Part model, mm, in its own coordinate system. A direction names the side the tool comes from. Round coordinates to 2 decimals unless told otherwise and drop trailing zeros. Order: outer loops, then holes, each group sorted by start corner. A loop starts at its lowest first (then second) coordinate and runs counter-clockwise, first axis right, second up. Notation, with made-up numbers: M 55.5,17 L 94.5,17 A11 ccw 94.5,26 Z; hole C 82,17 d4. An arc over 180 degrees is marked long. Write each question's results on one line, items separated by ' | '. Start each with the question number.
1. Two-plate mould, pull along Z, no slides. Class faces 6 (the face through (-74.289, -12.325, -74.196)), 7 (the face through (64, 0, 16)), 8 (the face through (77, 2, -1)): +Z half, -Z half, draft (parallel to the pull), parting line (faces both ways), or undercut.
2. Band-saw the part on C-C, the plane y = -59.5. List the corners of the cut face in (x, z), then the cut area to 3 significant figures.
3. Band-saw the part on A-A, the plane x = 0. List the corners of the cut face in (y, z).
4. Drop flat-ended pins along their axis: pin 1 Ø2 at (y, z) = (-39.5, 18) entering from +X; pin 2 Ø1.6 at (y, z) = (-7.5, 70.5) entering from -X; pin 3 Ø1 at (y, z) = (-13, 71) entering from +X. Give the stop position or say it passes through.
5. Probe L1, parallel to Z at x = 0, y = 1; L2, parallel to Z at x = 0, y = -49.5; L3, parallel to Z at x = 52.5, y = -4. List the from-to ranges inside material, lowest first. Write a range as [from, to].
6. Band-saw the part on B-B, the plane z = 0. List the corners of the cut face in (x, y).
7. Which spindle directions (+Z, -Z, +X, -X, +Y, -Y) get a long thin tool onto all of the face, cutting with end or side? Do faces 1 (the face through (-74.196, -12.325, 74.289)), 2 (the face through (74.289, -12.325, 74.196)), 3 (the face through (1, -12, 76)), 4 (the face through (62.475, -32.045, 19.674)), 5 (the face through (-1, -12, -76)). Say none if no direction does.
```python
from build123d import *

# Parameters (mm, degrees)
F0_W     = 154
F0_H     = 154
F1_DEPTH = 4
F3_DEPTH = 25
F4_R     = 65.5
F4_R_2   = 61.5
F5_DEPTH = 65
F6_DEPTH = 88.2


# Not quite as in the source:
# - ends of sketch curves that miss each other by under 0.0002 mm in the source are joined


with BuildPart() as f1:
    # F0 (on Front) → F1 (new body)
    with BuildSketch(Plane.XZ):
        Rectangle(F0_W, F0_H)
    extrude(amount=-F1_DEPTH)

    # F2 (on face) → F3 (join)
    with BuildSketch(Plane.XZ):
        with BuildLine():
            ThreePointArc((-76, -70), (-74.2426406871, -74.2426406871), (-70, -76))
            Line((-70, -76), (70, -76))
            ThreePointArc((70, -76), (74.2426406871, -74.2426406871), (76, -70))
            Line((76, -70), (76, 70))
            ThreePointArc((76, 70), (74.2426406871, 74.2426406871), (70, 76))
            Line((70, 76), (-70, 76))
            ThreePointArc((-70, 76), (-74.2426406871, 74.2426406871), (-76, 70))
            Line((-76, 70), (-76, -70))
        make_face()
        Polygon((-71.9999969006, 71.9999969006), (-70, 71.9999969006), (70, 72), (71.9999969006, 71.9999969006), (71.9999969006, 70), (72, -70), (71.9999969006, -71.9999969006), (70, -71.9999969006), (-70, -72), (-71.9999969006, -71.9999969006), (-71.9999969006, -70), (-72, 70), align=None, mode=Mode.SUBTRACT)
    extrude(amount=F3_DEPTH)

    # F4 (on face) → F5 (join)
    with BuildSketch(Plane.XZ):
        Circle(F4_R)
        Circle(F4_R_2, mode=Mode.SUBTRACT)
    extrude(amount=F5_DEPTH)

    # F6 (cut): a face of the model
    f6_faces = [f1.faces().sort_by_distance(p)[0] for p in [
        (0, 0, 0),
    ]]
    extrude(f6_faces, amount=-F6_DEPTH, mode=Mode.SUBTRACT)


solid = f1.part
```
Solution:
1) face 6: -Z half | face 7: undercut | face 8: draft
2) outline: C 0,0 d131; hole C 0,0 d123 | area: 1,600 mm^2
3) outline: M -65,-65.5 L 0,-65.5 L 0,-72 L -25,-72 L -25,-76 L 0,-76 L 0,-77 L 4,-77 L 4,-61.5 L -65,-61.5 Z; M -65,61.5 L 4,61.5 L 4,77 L 0,77 L 0,76 L -25,76 L -25,72 L 0,72 L 0,65.5 L -65,65.5 Z
4) pin 1: x = 63.26 | pin 2: x = -76 | pin 3: x = 75.98
5) L1: [-77, -61.5], [61.5, 77] | L2: [-65.5, -61.5], [61.5, 65.5] | L3: [-76, -72], [-39.17, -32.03], [32.03, 39.17], [72, 76]
6) outline: M -77,0 L -76,0 L -76,-25 L -72,-25 L -72,0 L -65.5,0 L -65.5,-65 L -61.5,-65 L -61.5,4 L -77,4 Z; M 61.5,-65 L 65.5,-65 L 65.5,0 L 72,0 L 72,-25 L 76,-25 L 76,0 L 77,0 L 77,4 L 61.5,4 Z
7) face 1: +Z, -X, -Y | face 2: +Z, +X, -Y | face 3: +Z, +X, -X, -Y | face 4: -Y | face 5: -Z, +X, -X, -Y
